from build123d import *

# Parameters (mm, degrees)
SKETCH1_R           = 6
BOSS_EXTRUDE1_DEPTH = 2.8
CHAMFER1_SIZE       = 0.859491926
CHAMFER1_SIZE_2     = 7
FILLET4_R           = 5
FILLET5_R           = 0.5
FILLET10_R          = 5
FILLET11_R          = 8


with BuildPart() as part:
    # Sketch1 → Boss-Extrude1 (new body)
    with BuildSketch(Plane(origin=(0, 0, 0), x_dir=(1, 0, 0), z_dir=(0, 1, 0))):
        Polygon((-9, 10), (-6, 13), (45, -4), (4, -9), (-6, -9), (-7.660869565, -2), (-15.8, 5.2), (-15.8, 8.7), (-9, 8.7), align=None)
        with Locations(Location((0, 0, 0), (0, 0, 270))):
            Circle(SKETCH1_R, mode=Mode.SUBTRACT)
    extrude(amount=BOSS_EXTRUDE1_DEPTH)

    # Chamfer1
    # the kernel refuses this chamfer: 7, 0.859491926 mm, written as the material it takes off along each edge
    with BuildSketch(Plane(origin=(-15.8, -18.194982295, -8.7), x_dir=(-0.29696840376135825, 0, 0.9548873060039236), z_dir=(0, 1, 0))) as chamfer1_piece_1_section:
        Polygon((CHAMFER1_SIZE * 0.95488730636, CHAMFER1_SIZE * 0.296968403872), (-CHAMFER1_SIZE_2 * 0.296968403761, CHAMFER1_SIZE_2 * 0.954887306004), (0, 0), align=None)
    chamfer1_piece_1 = extrude(amount=39.18996459, mode=Mode.PRIVATE)
    chamfer1_piece_1 = split(chamfer1_piece_1, bisect_by=Plane(origin=(-9, 1.4, -8.488844691), z_dir=(-1, 0, 0)), keep=Keep.TOP, mode=Mode.PRIVATE)
    add(chamfer1_piece_1, mode=Mode.SUBTRACT)

    # Fillet4
    # the kernel refuses this fillet: 5 mm, written as the material it adds along each edge
    with BuildSketch(Plane(origin=(-9, 0, -8.675443088), x_dir=(-0.9925461516413187, 0, 0.12186934340517559), z_dir=(0, 1, 0))) as fillet4_piece_1:
        with BuildLine():
            CenterArc((3.217696086, -5), FILLET4_R, 90, 42.518155203)
            Line((-0.161422881, -1.314683866), (-0.229005261, -1.240977543))
            ThreePointArc((-0.229005261, -1.240977543), (-0.179966056, -0.645154999), (-0.099254615, 0.012186934))
            Line((-0.099254615, 0.012186934), (0, 0.1))
            Line((0, 0.1), (3.217696086, 0.1))
            Line((3.217696086, 0.1), (3.217696086, 0))
        make_face()
    extrude(amount=2.8)

    # Fillet5
    fillet5_edges = [part.edges().sort_by_distance(p)[0] for p in [
        (-15.8, 1.4, -7.840508074),
    ]]
    fillet(fillet5_edges, radius=FILLET5_R)

    # Fillet10
    fillet10_edges = [part.edges().sort_by_distance(p)[0] for p in [
        (-7.660869565, 1.4, 2),
    ]]
    fillet(fillet10_edges, radius=FILLET10_R)

    # Fillet11
    fillet11_edges = [part.edges().sort_by_distance(p)[0] for p in [
        (-6, 1.4, 9),
    ]]
    fillet(fillet11_edges, radius=FILLET11_R)


solid = part.part
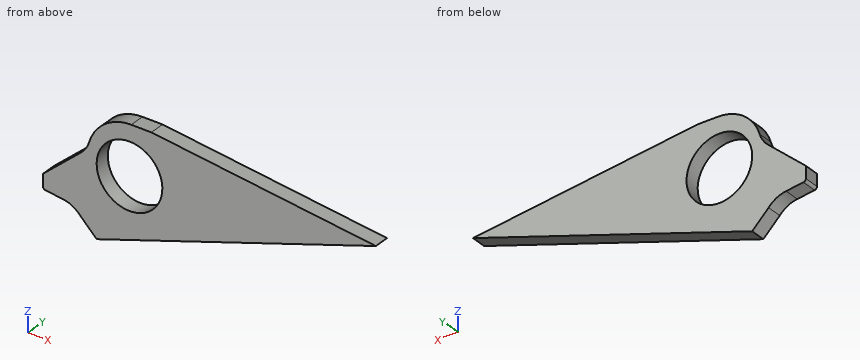
Can you work these out from the model? Positions are in its coordinate system, mm. Round coordinates to 2 decimals unless told otherwise and drop trailing zeros. Order: outer loops, then holes, each group sorted by start corner. A loop starts at its lowest first (then second) coordinate and runs counter-clockwise, first axis right, second up. Notation, with made-up numbers: (61, 83.5) -> (119, 83.5) arc R26 ccw to (119, 118.5) -> close; hole circle Ø5 at (21, 69.5). An arc over 180 degrees is marked (long way). Write each question's results on one line, items separated by ' | '. Start each with the question number.
Item 1: Please list where these lines run through material, in increasing order: L1, parallel to Z at x = 11, y = 0.8; L2, parallel to Z at x = 10, y = 2.1.
Item 2: If we section it at B-B, the plane x = 29.5: Write out the boundary of the cut face in (y, z).
Item 3: If we section it at C-C, the plane z = -10.75: Write out the boundary of the cut face in (x, y), then the cut area to 3 significant figures.
Item 4: If we section it at A-A, the plane z = 2.25: Write out the boundary of the cut face in (x, y).
Item 5: Will these pins go through, and if not, where does the flat tip stop? pin 1 (6 mm diameter, centred on x = 21, z = -7.5, fed in from -Y); pin 2 (1.5 mm diameter, centred on y = 2, z = -3, fed in from -X); pin 3 (6 mm diameter, centred on x = 7, z = -10, fed in from +Y).
Results:
1) L1: z = -7.33 to 8.15 | L2: z = -7.67 to 8.27
2) outline: (0, -1.17) -> (2.8, -1.17) -> (2.8, 5.89) -> (0, 5.89) -> close
3) outline: (-8.25, 0) -> (0.75, 0) -> (0.75, 2.8) -> (-8.25, 2.8) -> close | area: 25.2 mm2
4) outline: (-7.8, 0) -> (-5.56, 0) -> (-5.56, 2.8) -> (-7.8, 2.8) -> close; (5.56, 0) -> (39.75, 0) -> (39.75, 2.8) -> (5.56, 2.8) -> close
5) pin 1: passes through | pin 2: stops at x = -14.16 | pin 3: stops at y = 2.8
